Could you check a few things on this model? Use its own coordinates, in mm. A direction names the side the tool comes from. Give positions to 0.01 mm unless a question says otherwise; leave off trailing zeros. Write each loop counter-clockwise with the first axis right and the second up, starting at its lowest first coordinate (ties: lowest second). Pieces come first, ordered by that corner, then holes. Notation, with made-up numbers: (23.5, 65.25) - (58.5, 65.25) arc R26 cw to (58.5, 99.25) - close; hole circle Ø8 at (0.25, -5). An arc over 180 degrees is marked (long way). Write item = value, one per line.
from build123d import *

# Parameters (mm, degrees)
F1_DEPTH      = 3
F2_R          = 1.5
F2_W          = 4
F2_H          = 4
F3_DEPTH      = 13.5
F3_DEPTH_BACK = 9.5
F4_DEPTH      = 14.5
F5_DEPTH      = 8.5
F5_DEPTH_BACK = 4.5
F6_R          = 1
F9_DEPTH      = 1


with BuildPart() as f1:
    # F0 (on Top) → F1 (new body)
    with BuildSketch(Plane.XY):
        with BuildLine():
            Line((30.5, 27.5), (-30.5, 27.5))
            ThreePointArc((-30.5, 27.5), (-32.9748737342, 26.4748737342), (-34, 24))
            Line((-34, 24), (-34, -24))
            ThreePointArc((-34, -24), (-32.9748737342, -26.4748737342), (-30.5, -27.5))
            Line((-30.5, -27.5), (30.5, -27.5))
            ThreePointArc((30.5, -27.5), (32.9748737342, -26.4748737342), (34, -24))
            Line((34, -24), (34, 24))
            ThreePointArc((34, 24), (32.9748737342, 26.4748737342), (30.5, 27.5))
        make_face()
    extrude(amount=F1_DEPTH)

    # F2 (on Right) → F3 (join, two sides)
    with BuildSketch(Plane.YZ) as f3_sk:
        with BuildLine():
            Line((9.0669872981, 10.75), (4.5925227119, 3))
            Line((4.5925227119, 3), (21, 3))
            Line((21, 3), (21, 5.0505102572))
            ThreePointArc((21, 5.0505102572), (21.7267021942, 8.8558735008), (18.5, 11))
            Line((18.5, 11), (9.5, 11))
            ThreePointArc((9.5, 11), (9.25, 10.9330127019), (9.0669872981, 10.75))
        make_face()
        with Locations((18.5, 7.5)):
            Circle(F2_R, mode=Mode.SUBTRACT)
        with Locations((11.5, 8.5)):
            Rectangle(F2_W, F2_H, mode=Mode.SUBTRACT)
        with Locations((11.5, 8.5)):
            Rectangle(F2_W, F2_H)
    extrude(amount=F3_DEPTH)
    extrude(f3_sk.sketch, amount=-F3_DEPTH_BACK)

    # F2 (on Right) → F4 (join, through all)
    with BuildSketch(Plane.YZ):
        with Locations((11.5, 8.5)):
            Rectangle(F2_W, F2_H)
    extrude(amount=-F4_DEPTH)

    # F2 (on Right) → F5 (cut, two sides)
    with BuildSketch(Plane.YZ) as f5_sk:
        with BuildLine():
            Line((9.0669872981, 10.75), (4.5925227119, 3))
            Line((4.5925227119, 3), (21, 3))
            Line((21, 3), (21, 5.0505102572))
            ThreePointArc((21, 5.0505102572), (21.7267021942, 8.8558735008), (18.5, 11))
            Line((18.5, 11), (9.5, 11))
            ThreePointArc((9.5, 11), (9.25, 10.9330127019), (9.0669872981, 10.75))
        make_face()
        with Locations((18.5, 7.5)):
            Circle(F2_R, mode=Mode.SUBTRACT)
        with Locations((11.5, 8.5)):
            Rectangle(F2_W, F2_H, mode=Mode.SUBTRACT)
        with Locations((11.5, 8.5)):
            Rectangle(F2_W, F2_H)
    extrude(amount=F5_DEPTH, mode=Mode.SUBTRACT)
    extrude(f5_sk.sketch, amount=-F5_DEPTH_BACK, mode=Mode.SUBTRACT)

    # F6
    f6_edges = [f1.edges().sort_by_distance(p)[0] for p in [
        (0, -27.5, 0),
        (0, -27.5, 3),
    ]]
    fillet(f6_edges, radius=F6_R)

    # F8 (on face) → F9 (cut)
    with BuildSketch(Plane(origin=(0, 0, 0), x_dir=(1, 0, 0), z_dir=(0, 0, -1))):
        with BuildLine():
            Line((19.6177823817, -4.8641717246), (21.0291530011, -3.9822494804))
            ThreePointArc((21.0291530011, -3.9822494804), (21.1585557306, -3.6451438448), (20.8701772218, -3.4278350515))
            Line((20.8701772218, -3.4278350515), (11.0740224249, -3.4278350515))
            ThreePointArc((11.0740224249, -3.4278350515), (10.7856439161, -3.2105262583), (10.9150466456, -2.8734206227))
            Line((10.9150466456, -2.8734206227), (24.1127514461, 5.3734206227))
            ThreePointArc((24.1127514461, 5.3734206227), (24.2421541756, 5.7105262583), (23.9537756668, 5.9278350515))
            Line((23.9537756668, 5.9278350515), (7.7590025694, 5.9278350515))
            ThreePointArc((7.7590025694, 5.9278350515), (5.8295410786, 5.6566669231), (4.0495677197, 4.8641717246))
            Line((4.0495677197, 4.8641717246), (2.1580967416, 3.6822494804))
            ThreePointArc((2.1580967416, 3.6822494804), (2.0286940121, 3.3451438448), (2.3170725209, 3.1278350515))
            Line((2.3170725209, 3.1278350515), (12.1132273178, 3.1278350515))
            ThreePointArc((12.1132273178, 3.1278350515), (12.4016058266, 2.9105262583), (12.2722030971, 2.5734206227))
            Line((12.2722030971, 2.5734206227), (-0.4454013447, -5.3734206227))
            ThreePointArc((-0.4454013447, -5.3734206227), (-0.5748040742, -5.7105262583), (-0.2864255655, -5.9278350515))
            Line((-0.2864255655, -5.9278350515), (15.908347532, -5.9278350515))
            ThreePointArc((15.908347532, -5.9278350515), (17.8378090227, -5.6566669231), (19.6177823817, -4.8641717246))
        make_face()
        with BuildLine():
            Line((-5.1827407197, -4.560267917), (-3.4575505927, -3.4822494804))
            ThreePointArc((-3.4575505927, -3.4822494804), (-3.3281478632, -3.1451438448), (-3.616526372, -2.9278350515))
            Line((-3.616526372, -2.9278350515), (-6.7218778514, -2.9278350515))
            Line((-6.7218778514, -2.9278350515), (-7.5220451159, -3.4278350515))
            Line((-7.5220451159, -3.4278350515), (-19.2220485259, -3.4278350515))
            ThreePointArc((-19.2220485259, -3.4278350515), (-19.4568309729, -3.3145894425), (-19.5143595453, -3.0603497352))
            Line((-19.5143595453, -3.0603497352), (-19.3168125364, -2.2046796322))
            ThreePointArc((-19.3168125364, -2.2046796322), (-19.211255908, -2.0373825014), (-19.024501517, -1.9721649485))
            Line((-19.024501517, -1.9721649485), (-7.3452009568, -1.9721649485))
            ThreePointArc((-7.3452009568, -1.9721649485), (-7.0339436385, -1.8634690269), (-6.8580159244, -1.5846404756))
            Line((-6.8580159244, -1.5846404756), (-6.5117136377, -0.0846404756))
            ThreePointArc((-6.5117136377, -0.0846404756), (-6.6075945917, 0.3390923699), (-6.9988986701, 0.5278350515))
            Line((-6.9988986701, 0.5278350515), (-18.3088101245, 0.5278350515))
            ThreePointArc((-18.3088101245, 0.5278350515), (-18.5435925715, 0.6410806606), (-18.6011211439, 0.8953203678))
            Line((-18.6011211439, 0.8953203678), (-18.1393847617, 2.8953203678))
            ThreePointArc((-18.1393847617, 2.8953203678), (-18.0338281332, 3.0626174986), (-17.8470737422, 3.1278350515))
            Line((-17.8470737422, 3.1278350515), (-5.8134825092, 3.1278350515))
            Line((-5.8134825092, 3.1278350515), (-5.0133152446, 2.6278350515))
            Line((-5.0133152446, 2.6278350515), (-1.9079637652, 2.6278350515))
            ThreePointArc((-1.9079637652, 2.6278350515), (-1.6195852564, 2.8451438448), (-1.748987986, 3.1822494804))
            Line((-1.748987986, 3.1822494804), (-4.4406262286, 4.8641717246))
            ThreePointArc((-4.4406262286, 4.8641717246), (-6.2205995875, 5.6566669231), (-8.1500610782, 5.9278350515))
            Line((-8.1500610782, 5.9278350515), (-20.6720310554, 5.9278350515))
            ThreePointArc((-20.6720310554, 5.9278350515), (-21.9170603287, 5.4930513653), (-22.620771185, 4.3777371602))
            Line((-22.620771185, 4.3777371602), (-23.3027861367, 1.4236058509))
            ThreePointArc((-23.3027861367, 1.4236058509), (-23.2457131813, 0.5594631094), (-22.7204795121, -0.1291075788))
            ThreePointArc((-22.7204795121, -0.1291075788), (-22.5997954695, -0.4176373884), (-22.8013911757, -0.6567466947))
            ThreePointArc((-22.8013911757, -0.6567466947), (-23.6483083742, -1.208565733), (-24.1172110997, -2.1040562277))
            Line((-24.1172110997, -2.1040562277), (-24.5757966488, -4.09040847))
            ThreePointArc((-24.5757966488, -4.09040847), (-24.2881537869, -5.3616070065), (-23.1142415516, -5.9278350515))
            Line((-23.1142415516, -5.9278350515), (-9.9520140978, -5.9278350515))
            ThreePointArc((-9.9520140978, -5.9278350515), (-7.4712778955, -5.579190315), (-5.1827407197, -4.560267917))
        make_face()
    extrude(amount=-F9_DEPTH, mode=Mode.SUBTRACT)


solid = f1.part
1. If we section it at A-A, the plane x = -29: Please give me the cut outline in (y, z), and give its area (3 significant figures).
Filled sheet:
outline = (-27.5, 1) arc R1 ccw to (-26.5, 0) - (26.5, 0) arc R1 ccw to (27.5, 1) - (27.5, 2) arc R1 ccw to (26.5, 3) - (-26.5, 3) arc R1 ccw to (-27.5, 2) - close
area = 164 mm2
2. Which directions (+Z, -Z, +X, -X, +Y, -Y) give clear straight access to the entire face, cutting with the end or side of a thin tool? Please do faces 1 (the face through (8.5, 13, 7)), 2 (the face through (-14.5, 11, 9)), 3 (the face through (11, 21, 4)), 4 (the face through (6.002, 1.344, 0.493)), 5 (the face through (13.5, 13, 7)).
Filled sheet:
face_1 = +Z, +Y, -Y
face_2 = +Z, -X, +Y, -Y
face_3 = +X, -X, +Y
face_4 = -Z
face_5 = +Z, +X, +Y, -Y
3. For pin 1 (1.6 mm diameter, centred on x = -8, z = 3.5, fed in from +Y); pin 2 (1.1 mm diameter, centred on x = -12, z = 0.5, fed in from +Y); pin 3 (3 mm diameter, centred on y = 11, z = 8, fed in from -X); pin 4 (4 mm diameter, centred on x = 26, y = 15, fed in from +Z), each with a flat end and sliding along its axis, tell me the tip position at first contact or that it passes through.
Filled sheet:
pin_1 = 27.21
pin_2 = 27.5
pin_3 = -14.5
pin_4 = 3
4. If we section it at C-C, the plane z = 7.5: Please give me the cut outline in (x, y), and give its area (3 significant figures).
Filled sheet:
outline = (-14.5, 9.5) - (-9.5, 9.5) - (-9.5, 7.19) - (-4.5, 7.19) - (-4.5, 17) - (-9.5, 17) - (-9.5, 13.5) - (-14.5, 13.5) - close; (-9.5, 20) - (-4.5, 20) - (-4.5, 22) - (-9.5, 22) - close; (8.5, 7.19) - (13.5, 7.19) - (13.5, 17) - (8.5, 17) - close; (8.5, 20) - (13.5, 20) - (13.5, 22) - (8.5, 22) - close
area = 138 mm2
5. I need wall thicknesses on line 1 (X direction, y = 9, z = 8.5); line 2 (Z direction, x = 11.7, y = 18.5); line 3 (Z direction, x = -29.5, y = -21.5). Which ranges of each line are inside material? Lowest first, please.
Filled sheet:
line_1 = -9.5 to -4.5, 8.5 to 13.5
line_2 = 0 to 6, 9 to 11
line_3 = 0 to 3
6. Thinking about a two-plate mould opening in Y: for faces 6 (the face through (-7.51, 5.59, 0.49)), 7 (the face through (-12, 9.5, 8)), 8 (the face through (-12, 11, 6.5)), which applies, pulls with the +Y half, pulls with the -Y half, needs draft (parallel to the pull), parting line crosses it, or undercut?
Filled sheet:
face_6 = undercut
face_7 = pulls with the -Y half
face_8 = needs draft
7. If we section it at B-B, the plane y = -12.5: Please give me the cut outline in (x, z).
Filled sheet:
outline = (-34, 1) arc R1 ccw to (-33, 0) - (33, 0) arc R1 ccw to (34, 1) - (34, 2) arc R1 ccw to (33, 3) - (-33, 3) arc R1 ccw to (-34, 2) - close
